Study the drawing (mm; zero at the part's minimum x, y, z) and answer. Give positions to 0.01 mm unless a question says otherwise; leave off trailing zeros. Write each loop counter-clockwise with the first axis right and the second up, starting at its lowest first coordinate (ties: lowest second). Pieces come first, ordered by that corner, then holes.
1) Find section B-B (y = 2.45). Determine the outline of the cut face in (x, z).
2) Find section C-C (x = 17). Determine the outline of the cut face in (y, z).
3) Find section A-A (x = 24.56). Determine the outline of the cut face in (y, z).
4) Straight lines are drawn through the part: probe 1 along X at (y, z) = (1.45, 2.54); probe 2 along Z at (x, y) = (25.5, 1.9); probe 3 along Y at (x, z) = (6.5, 18). For each, find the intervals that lie inside material, in ascending order.
5) Determine the mould class of the marked faces 1, 2, 3 and 4 for opening direction Z: pulls with the +Z half, pulls with the -Z half, needs draft (parallel to the pull), parting line crosses it, or undercut.
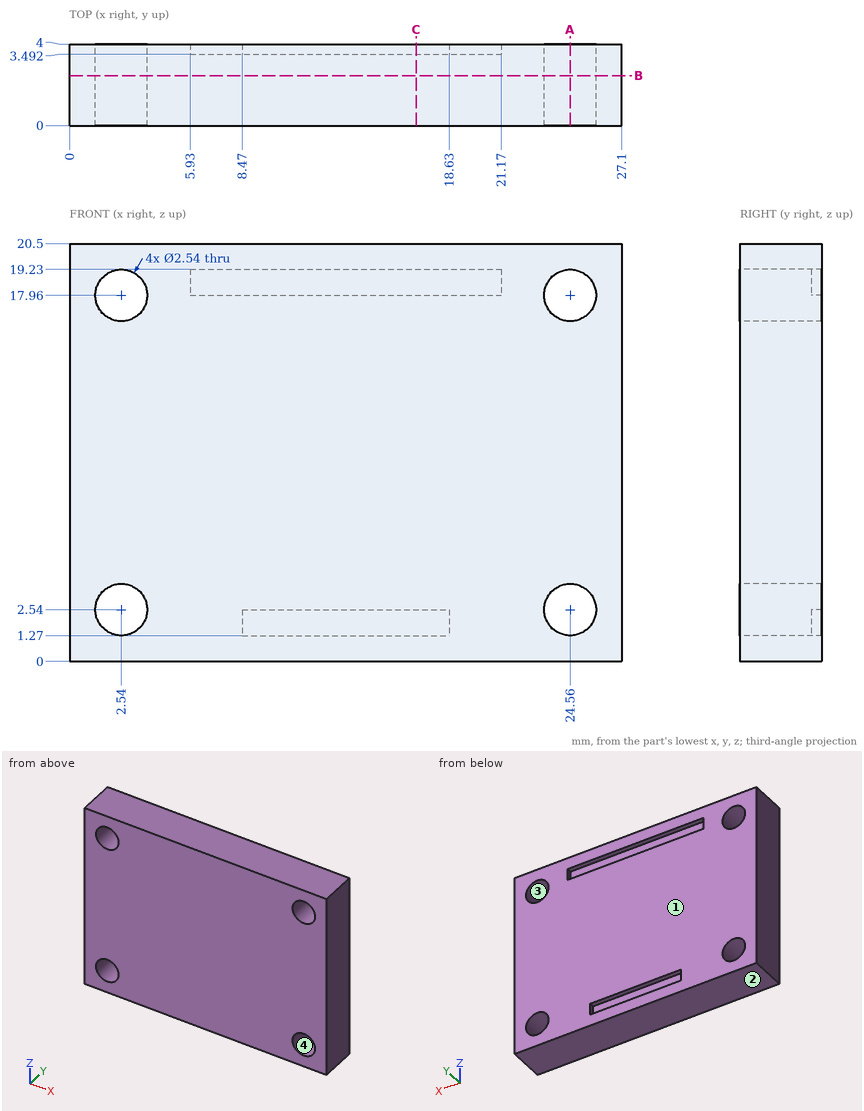
Results:
1. outline: (0, 0) - (27.1, 0) - (27.1, 20.5) - (0, 20.5) - close; hole circle Ø2.54 at (2.54, 2.54); hole circle Ø2.54 at (2.54, 17.96); hole circle Ø2.54 at (24.56, 2.54); hole circle Ø2.54 at (24.56, 17.96)
2. outline: (0, 0) - (4, 0) - (4, 1.27) - (3.49, 1.27) - (3.49, 2.54) - (4, 2.54) - (4, 17.96) - (3.49, 17.96) - (3.49, 19.23) - (4, 19.23) - (4, 20.5) - (0, 20.5) - close
3. outline: (0, 0) - (4, 0) - (4, 1.27) - (0, 1.27) - close; (0, 3.81) - (4, 3.81) - (4, 16.69) - (0, 16.69) - close; (0, 19.23) - (4, 19.23) - (4, 20.5) - (0, 20.5) - close
4. probe 1: x = 0 to 1.27, 3.81 to 23.29, 25.83 to 27.1
4. probe 2: z = 0 to 1.69, 3.39 to 17.11, 18.81 to 20.5
4. probe 3: y = 0 to 3.49
5. face 1: needs draft
5. face 2: pulls with the -Z half
5. face 3: undercut
5. face 4: undercut
